Autodesk Inventor part; units mm, degrees
ref_plane "YZ Plane" through (0, 0, 0) normal (1, 0, 0) x (0, 1, 0)
ref_plane "XZ Plane" through (0, 0, 0) normal (0, 1, 0) x (-1, 0, 0)
ref_plane "XY Plane" through (0, 0, 0) normal (0, 0, 1) x (1, 0, 0)
sketch "Sketch1" plane through (0, 0, 0) normal (1, 0, 0) x (0, 1, 0)
  line L0 (0, 0) -> (25.4, 0)
  line L1 (25.4, 0) -> (25.4, 3.175)
  line L2 (25.4, 3.175) -> (3.175, 3.175)
  line L3 (3.175, 3.175) -> (3.175, 50.8)
  line L4 (3.175, 50.8) -> (0, 50.8)
  line L5 (0, 50.8) -> (0, 0)
  dimension "d0" = 25.4
  dimension "d1" = 3.175
  dimension "d2" = 22.225
  dimension "d3" = 47.625
extrude "Extrusion1" add sketch "Sketch1" along normal blind 50.8
sketch "Sketch2" plane through (0, 3.175, 3.175) normal (0, 0, 1) x (1, 0, 0)
  circle A0 centre (12.7, 9.525) radius 3.175
  circle A1 centre (38.1, 9.525) radius 3.175
  line L0 (0, 22.225) -> (50.8, 22.225)
  line L1 (50.8, 22.225) -> (50.8, 0)
  line L2 (0, 22.225) -> (0, 0)
  point P0 (0, -3.175)
  dimension "d6" = 6.35
  dimension "d7" = 12.7
  dimension "d8" = 12.7
  dimension "d9" = 12.7
  dimension "d10" = 12.7
extrude "Extrusion2" cut sketch "Sketch2" against normal blind 3.175
sketch "Sketch3" plane through (0, 3.175, 50.8) normal (0, 1, 0) x (1, 0, 0)
  circle A0 centre (12.7, 12.7) radius 3.175
  circle A1 centre (12.7, 38.1) radius 3.175
  line L0 (0, 0) -> (50.8, 0)
  line L1 (0, 47.625) -> (0, 0)
  point P0 (0, 50.8)
  dimension "d13" = 6.35
  dimension "d14" = 6.35
  dimension "d15" = 12.7
  dimension "d16" = 12.7
  dimension "d17" = 12.7
  dimension "d18" = 38.1
extrude "Extrusion3" cut sketch "Sketch3" against normal blind 3.175
properties part number "angle gusset"
Source: CAD feature listing. Evaluate the final solid. Frame: model axes, mm. Give positions to 0.01 mm unless a question says otherwise; leave off trailing zeros. Order: outer loops, then holes, each group sorted by start corner. A loop starts at its lowest first (then second) coordinate and runs counter-clockwise, first axis right, second up. Notation, with made-up numbers: (9, -4.5) -> (38, -4.5) arc R26 ccw to (38, 34.5) -> close; hole circle Ø7 at (65.25, -3.75). An arc over 180 degrees is marked (long way). Write item = value, one per line.
Item 1: Section query B-B (y = 12.7). Output: boundary loops of the cut face in (x, z) (3 decimals), then the cut area to 3 significant figures.
Check result:
outline = (0, 0) -> (9.525, 0) -> (9.525, 3.175) -> (0, 3.175) -> close; (15.875, 0) -> (34.925, 0) -> (34.925, 3.175) -> (15.875, 3.175) -> close; (41.275, 0) -> (50.8, 0) -> (50.8, 3.175) -> (41.275, 3.175) -> close
area = 121 mm²
Item 2: Ray query, probe 1 along Z at (x, y) = (12.7, 2.15) (3 decimals); probe 2 along X at (y, z) = (2.15, 12.7) (3 decimals); probe 3 along Y at (x, z) = (38, 1). Return the intervals inside material, ascending.
Check result:
probe_1 = 0 to 9.525, 15.875 to 34.925, 41.275 to 50.8
probe_2 = 0 to 9.525, 15.875 to 50.8
probe_3 = 0 to 9.53, 15.87 to 25.4
Item 3: Section query C-C (z = 12.7). Output: boundary loops of the cut face in (x, y) (3 decimals), then the cut area to 3 significant figures.
Check result:
outline = (0, 0) -> (9.525, 0) -> (9.525, 3.175) -> (0, 3.175) -> close; (15.875, 0) -> (50.8, 0) -> (50.8, 3.175) -> (15.875, 3.175) -> close
area = 141 mm²
Item 4: Contact query for flat-ended pins moving along their axis: pin 1 (1.5 mm diameter, centred on x = 15.5, y = 11, fed in from +Z) (3 decimals); pin 2 (1.5 mm diameter, centred on x = 12.5, z = 27, fed in from +Y) (3 decimals). Output: stop coordinate, or through.
Check result:
pin_1 = 3.175
pin_2 = 3.175
Item 5: Section query D-D (x = 38.1). Output: boundary loops of the cut face in (y, z) (3 decimals).
Check result:
outline = (0, 0) -> (9.525, 0) -> (9.525, 3.175) -> (3.175, 3.175) -> (3.175, 50.8) -> (0, 50.8) -> close; (15.875, 0) -> (25.4, 0) -> (25.4, 3.175) -> (15.875, 3.175) -> close
Item 6: Section query A-A (x = 12.7). Output: boundary loops of the cut face in (y, z) (3 decimals).
Check result:
outline = (0, 0) -> (9.525, 0) -> (9.525, 3.175) -> (3.175, 3.175) -> (3.175, 9.525) -> (0, 9.525) -> close; (0, 15.875) -> (3.175, 15.875) -> (3.175, 34.925) -> (0, 34.925) -> close; (0, 41.275) -> (3.175, 41.275) -> (3.175, 50.8) -> (0, 50.8) -> close; (15.875, 0) -> (25.4, 0) -> (25.4, 3.175) -> (15.875, 3.175) -> close
Item 7: Mould query, pull axis Z, two halves, no side actions, for faces 1 (the face through (25, 14, 3.175)), 2 (the face through (25, 3.175, 27)), 3 (the face through (12.29, 1.61, 34.95)). Classes: +Z half, -Z half, draft (parallel to the pull), parting line (faces both ways), or undercut.
Check result:
face_1 = +Z half
face_2 = draft
face_3 = undercut
